Part model, mm, in its own coordinate system. A direction names the side the tool comes from. Coordinates: 2 decimals unless noted, no trailing zeros. Loops run counter-clockwise (first coordinate to the right, second up) from the corner with the lowest first, then second, coordinate; pieces in that order, holes last. Notation, with made-up numbers: (3.5, 27) -> (53.5, 27) arc R8 ccw to (53.5, 31) -> close; hole circle Ø10 at (27.5, 46.5). An arc over 180 degrees is marked (long way). One line per item, written item: value. Start each with the question number.
from build123d import *

# Parameters (mm, degrees)
SKETCH1_W           = 57.15
SKETCH1_H           = 6.35
BOSS_EXTRUDE1_DEPTH = 76.2
SKETCH2_W           = 50.8
SKETCH2_H           = 3.175
CUT_EXTRUDE1_DEPTH  = 73.025
SKETCH4_R           = 1.25
CUT_EXTRUDE2_DEPTH  = 4.175


with BuildPart() as part:
    # Sketch1 → Boss-Extrude1 (new body)
    with BuildSketch(Plane(origin=(0, 0, 0), x_dir=(1, 0, 0), z_dir=(0, 1, 0))):
        Rectangle(SKETCH1_W, SKETCH1_H)
    extrude(amount=BOSS_EXTRUDE1_DEPTH)

    # Sketch2 → Cut-Extrude1 (cut)
    with BuildSketch(Plane(origin=(0, 76.2, 0), x_dir=(1, 0, 0), z_dir=(0, 1, 0))):
        with Locations((0, 1.5875)):
            Rectangle(SKETCH2_W, SKETCH2_H)
    extrude(amount=-CUT_EXTRUDE1_DEPTH, mode=Mode.SUBTRACT)

    # Sketch4 → Cut-Extrude2 (cut, through all)
    with BuildSketch(Plane(origin=(0, 0, 0), x_dir=(-1, 0, 0), z_dir=(0, 0, -1))):
        with Locations((-9.525, 66.675)):
            Circle(SKETCH4_R)
        with Locations((9.525, 66.675)):
            Circle(SKETCH4_R)
        with Locations((-15.875, 15.875)):
            Circle(SKETCH4_R)
        with Locations((15.875, 15.875)):
            Circle(SKETCH4_R)
    extrude(amount=-CUT_EXTRUDE2_DEPTH, mode=Mode.SUBTRACT)


solid = part.part
1) Probe line 1 (X direction, y = 70.5, z = -0.5) (3 decimals); line 2 (Z direction, x = -1, y = 17) (3 decimals). List the from-to ranges inside material, lowest first. Write a range as from..to.
2) Slice it at C-C (x = 23.5). Give the cut face in (y, z) (3 decimals).
3) Tool access for faces 1 (the flat face through (0, 40, 0)), 2 (the flat face through (28.575, 38, 0)): list every direction of +Z, -Z, +X, -X, +Y, -Y with a clear straight run to the whole face (end or side of a thin tool).
4) Slice it at B-B (y = 64). Give the cut face in (x, z) (3 decimals), then the cut area to 3 significant figures.
5) Pull direction X, two halves, no side cores. Call faces 3 (the flat face through (0, 38, 3.175)), 4 (the flat face through (-28.575, 38, 0)), 5 (the cylindrical face through (-16.547, 16.929, 1.565)): +X half, -X half, draft (parallel to the pull), parting line (faces both ways), or undercut.
6) Pin check, flat tips, straight feed: pin 1 Ø1.5 at (x, y) = (-13.5, 66) entering from -Z; pin 2 Ø1.6 at (x, z) = (12.5, -1) entering from +Y (3 decimals). Stop position of each tip, or through.
7) Slice it at A-A (z = -1.5). Give the cut face in (x, y) (3 decimals).
Check sheet entries:
1. line 1: x = -28.575..-25.4, 25.4..28.575
1. line 2: z = 0..3.175
2. outline: (0, -3.175) -> (3.175, -3.175) -> (3.175, 0) -> (76.2, 0) -> (76.2, 3.175) -> (0, 3.175) -> close
3. face 1: -Z, +Y
3. face 2: +Z, -Z, +X, +Y, -Y
4. outline: (-28.575, -3.175) -> (-25.4, -3.175) -> (-25.4, 0) -> (25.4, 0) -> (25.4, -3.175) -> (28.575, -3.175) -> (28.575, 3.175) -> (-28.575, 3.175) -> close
4. area: 202 mm^2
5. face 3: draft
5. face 4: -X half
5. face 5: undercut
6. pin 1: stops at z = 0
6. pin 2: stops at y = 3.175
7. outline: (-28.575, 0) -> (28.575, 0) -> (28.575, 76.2) -> (25.4, 76.2) -> (25.4, 3.175) -> (-25.4, 3.175) -> (-25.4, 76.2) -> (-28.575, 76.2) -> close
